Part print with two shaded views. Sizes in mm from the minimum x, y, z corner. A direction names the side the tool comes from. Give positions to 0.01 mm unless a question says otherwise; leave off trailing zeros. Order: outer loops, then holes, each group sorted by start corner. A loop starts at its lowest first (then second) coordinate and runs counter-clockwise, first axis right, second up. Notation, with made-up numbers: (-39, 49.25) -> (18, 49.25) arc R23 cw to (18, 77.25) -> close; hole circle Ø8 at (-11, 53). An arc over 180 degrees is marked (long way). Answer as CSV lines item,"result".
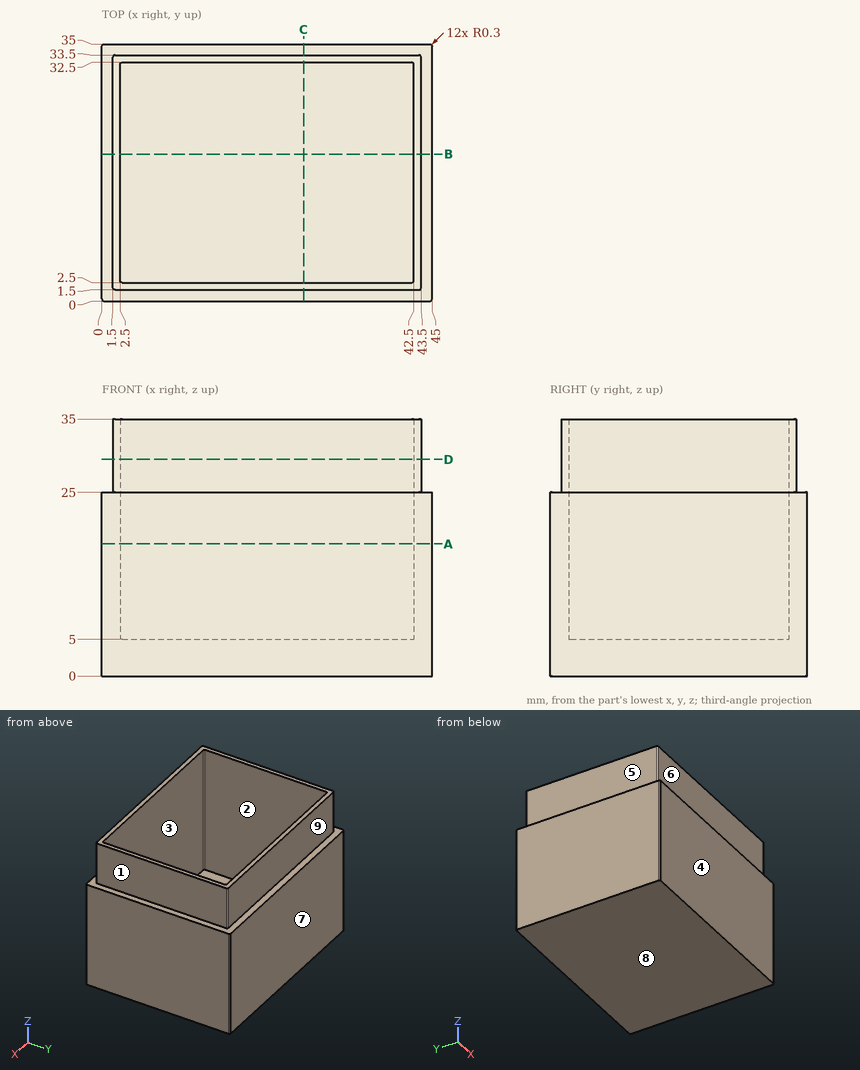
1) Band-saw the part on D-D, the plane z = 29.5. Write the cut outline in (x, y), then the cut area to 3 significant figures.
Data:
outline,"(1.5, 1.8) arc R0.3 ccw to (1.8, 1.5) -> (43.2, 1.5) arc R0.3 ccw to (43.5, 1.8) -> (43.5, 33.2) arc R0.3 ccw to (43.2, 33.5) -> (1.8, 33.5) arc R0.3 ccw to (1.5, 33.2) -> close; hole (2.5, 2.8) arc R0.3 ccw to (2.8, 2.5) -> (42.2, 2.5) arc R0.3 ccw to (42.5, 2.8) -> (42.5, 32.2) arc R0.3 ccw to (42.2, 32.5) -> (2.8, 32.5) arc R0.3 ccw to (2.5, 32.2) -> close"
area,"144 mm2"
2) Which spindle directions (+Z, -Z, +X, -X, +Y, -Y) get a long thin tool onto all of the face, cutting with end or side? Do the marked faces 5, 6, 7, 8 and 9. Say none if no direction does.
Data:
face 5,"+Z, -X, +Y, -Y"
face 6,"+Z, +X, -X, -Y"
face 7,"+Z, -Z, +X, -X, +Y"
face 8,"-Z, +X, -X, +Y, -Y"
face 9,"+Z, +X, -X, +Y"
3) Wall check: line 1 along X through (y, z) = (9, 29); line 2 along Y through (x, z) = (42, 8); line 3 along X through (y, z) = (25, 9). Give the ranges that are in metal, low to high. Write a range as [from, to].
Data:
line 1,"x = [1.5, 2.5], [42.5, 43.5]"
line 2,"y = [0, 2.5], [32.5, 35]"
line 3,"x = [0, 2.5], [42.5, 45]"
4) Band-saw the part on A-A, the plane z = 18. Write the cut outline in (x, y).
Data:
outline,"(0, 0.3) arc R0.3 ccw to (0.3, 0) -> (44.7, 0) arc R0.3 ccw to (45, 0.3) -> (45, 34.7) arc R0.3 ccw to (44.7, 35) -> (0.3, 35) arc R0.3 ccw to (0, 34.7) -> close; hole (2.5, 2.8) arc R0.3 ccw to (2.8, 2.5) -> (42.2, 2.5) arc R0.3 ccw to (42.5, 2.8) -> (42.5, 32.2) arc R0.3 ccw to (42.2, 32.5) -> (2.8, 32.5) arc R0.3 ccw to (2.5, 32.2) -> close"
5) Pin check, flat tips, straight feed: P1, Ø3, axis at x = 17, z = 28.5, coming from the +Y side; P2, Ø15, axis at x = 30, y = 20, coming from the +Z side; P3, Ø3, axis at y = 13, z = 30.5, coming from the -X side. Stop position of each tip, or through.
Data:
P1,"stops at y = 33.5"
P2,"stops at z = 5"
P3,"stops at x = 1.5"
6) Pull direction Y, two halves, no side cores. Call the marked faces 1, 2, 3 and 4: pulls with the +Y half, pulls with the -Y half, needs draft (parallel to the pull), parting line crosses it, or undercut.
Data:
face 1,"needs draft"
face 2,"undercut"
face 3,"undercut"
face 4,"pulls with the -Y half"
7) Band-saw the part on C-C, the plane x = 27.5. Write the cut outline in (y, z), then the cut area to 3 significant figures.
Data:
outline,"(0, 0) -> (35, 0) -> (35, 25) -> (33.5, 25) -> (33.5, 35) -> (32.5, 35) -> (32.5, 5) -> (2.5, 5) -> (2.5, 35) -> (1.5, 35) -> (1.5, 25) -> (0, 25) -> close"
area,"295 mm2"
8) Band-saw the part on B-B, the plane y = 20. Write the cut outline in (x, z).
Data:
outline,"(0, 0) -> (45, 0) -> (45, 25) -> (43.5, 25) -> (43.5, 35) -> (42.5, 35) -> (42.5, 5) -> (2.5, 5) -> (2.5, 35) -> (1.5, 35) -> (1.5, 25) -> (0, 25) -> close"
